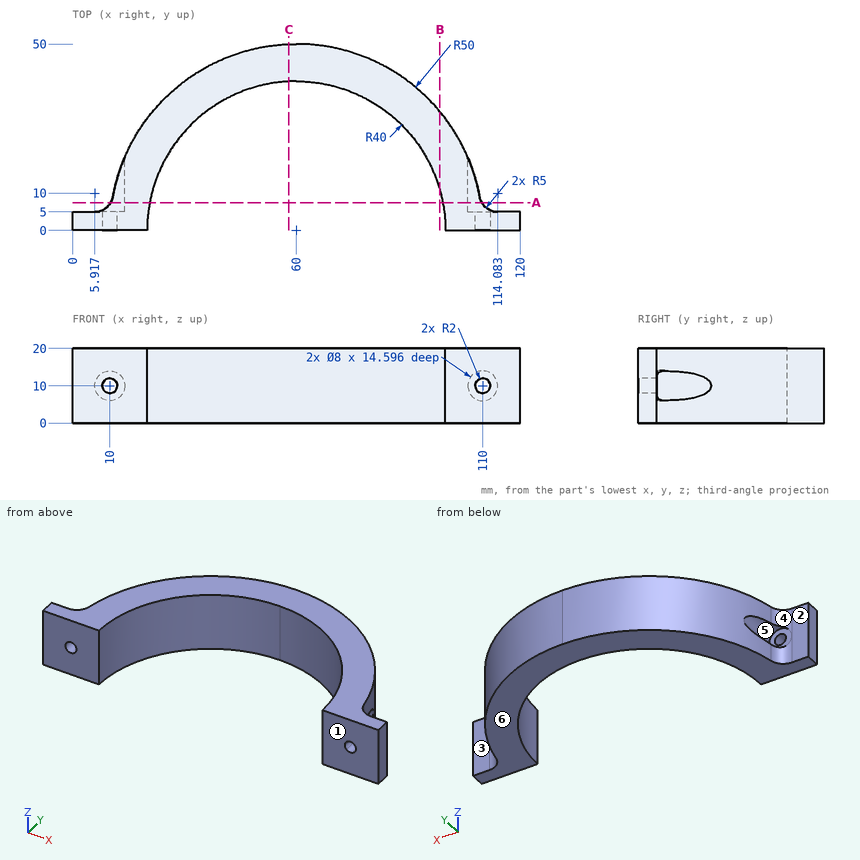
Geometry check sheet. Reference: drawing and pictorial views, mm from the part's lowest x, y, z. A direction names the side the tool comes from. Coordinates: 2 decimals unless noted, no trailing zeros. Loops run counter-clockwise (first coordinate to the right, second up) from the corner with the lowest first, then second, coordinate; pieces in that order, holes last.
1) Release check for a two-part mould opening along Z. For the marked faces 4, 5 and 6 record: released by +Z, released by -Z, zero draft, split by the parting line, or undercut.
2) Gauge pin test, flat ends, axial feed: pin 1 (4 mm diameter, centred on x = 10, z = 10.5, fed in from +Y); pin 2 (1 mm diameter, centred on y = 20.5, z = 17, fed in from +X); pin 3 (10 mm diameter, centred on y = 38.5, z = 15.5, fed in from -X); pin 4 (1.5 mm diameter, centred on x = 92, y = 20, fed in from -Z). Record the tip position at first contact, or that the pin passes through.
3) Sectioned sample at C-C (x = 58). Record the boundary of the cut face in (y, z), and give its area (3 significant figures).
4) Sectioned sample at A-A (y = 7.5). Record the boundary of the cut face in (x, z).
5) Material ranges on probe 1 along Y at (x, z) = (115, 10); probe 2 along X at (y, z) = (19, 7.5); probe 3 along X at (y, z) = (37, 13.5), recorded low to high.
6) Access from +Z, -Z, +X, -X, +Y, -Y to the whole of each face (thin tool, end or side, straight path). Record for the marked faces 1, 2 and 3.
7) Sectioned sample at B-B (x = 98.5). Record the boundary of the cut face in (y, z), and give its area (3 significant figures).
Check sheet entries:
1. face 4: zero draft
1. face 5: undercut
1. face 6: released by -Z
2. pin 1: stops at y = 5
2. pin 2: stops at x = 105.83
2. pin 3: stops at x = 22.88
2. pin 4: passes through
3. outline: (39.95, 0) - (49.96, 0) - (49.96, 20) - (39.95, 20) - close
3. area: 200 mm2
4. outline: (10.25, 0) - (20.71, 0) - (20.71, 20) - (10.25, 20) - (10.25, 13.99) arc R4 cw to (10.25, 6.01) - close; (99.29, 0) - (109.75, 0) - (109.75, 6.01) arc R4 cw to (109.75, 13.99) - (109.75, 20) - (99.29, 20) - close
5. probe 1: y = 0 to 5
5. probe 2: x = 13.75 to 24.8, 95.2 to 106.25
5. probe 3: x = 26.37 to 44.8, 75.2 to 93.63
6. face 1: +Z, -Z, +X, -X, -Y
6. face 2: +Z, -Z, -X, +Y
6. face 3: +Z, -Z, +X, +Y
7. outline: (10.85, 0) - (31.9, 0) - (31.9, 20) - (10.85, 20) - close
7. area: 421 mm2
